Geometry: final body of the model. Coordinates: model frame, mm. Face numbers are marked on the shaded views. A direction names the side the tool comes from. Round coordinates to 2 decimals unless told otherwise and drop trailing zeros. Write each loop counter-clockwise with the first axis right and the second up, starting at its lowest first coordinate (ties: lowest second). Pieces come first, ordered by that corner, then holes.
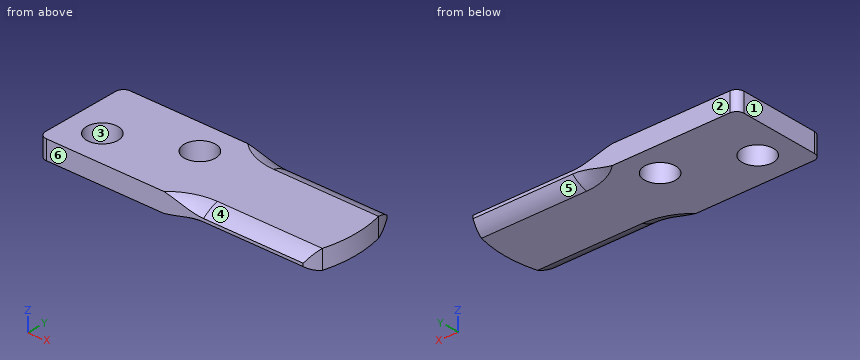
from build123d import *

# Parameters (mm, degrees)
F0_R     = 3.2512
F1_DEPTH = 3.9624


with BuildPart() as f1:
    # F0 (on Top) → F1 (new body)
    with BuildSketch(Plane.XY):
        with BuildLine():
            ThreePointArc((1.5875, 9.8425), (0.464968, 9.377532), (0, 8.255))
            Line((0, 8.255), (0, -8.255))
            ThreePointArc((0, -8.255), (0.464968, -9.377532), (1.5875, -9.8425))
            Line((1.5875, -9.8425), (26.001034, -9.8425))
            ThreePointArc((26.001034, -9.8425), (29.838111, -7.433166), (34.29, -6.5913))
            Line((34.29, -6.5913), (56.127475, -6.5913))
            ThreePointArc((56.127475, -6.5913), (56.9976, 0), (56.127475, 6.5913))
            Line((56.127475, 6.5913), (34.29, 6.5913))
            ThreePointArc((34.29, 6.5913), (29.838111, 7.433166), (26.001034, 9.8425))
            Line((26.001034, 9.8425), (1.5875, 9.8425))
        make_face()
        with Locations((7.0104, -2.8321)):
            Circle(F0_R, mode=Mode.SUBTRACT)
        with Locations((21.9964, 3.1623)):
            Circle(F0_R, mode=Mode.SUBTRACT)
        with BuildLine():
            Line((55.01309, 9.8425), (26.001034, 9.8425))
            ThreePointArc((26.001034, 9.8425), (29.838111, 7.433166), (34.29, 6.5913))
            Line((34.29, 6.5913), (56.127475, 6.5913))
            ThreePointArc((56.127475, 6.5913), (55.625336, 8.23577), (55.01309, 9.8425))
        make_face()
        with BuildLine():
            ThreePointArc((34.29, -6.5913), (29.838111, -7.433166), (26.001034, -9.8425))
            Line((26.001034, -9.8425), (55.01309, -9.8425))
            ThreePointArc((55.01309, -9.8425), (55.625336, -8.23577), (56.127475, -6.5913))
            Line((56.127475, -6.5913), (34.29, -6.5913))
        make_face()
    extrude(amount=F1_DEPTH)

    # F4: sweep along a path in F0
    with BuildLine(Plane.XY) as f4_path:
        Line((60.852341, 6.5913), (34.29, 6.5913))
        ThreePointArc((34.29, 6.5913), (29.838111, 7.433166), (26.001034, 9.8425))
    # F3 (on offset) → F4 (sweep, cut)
    with BuildSketch(Plane.YZ.offset(56.9976)):
        with BuildLine():
            Line((13.0175, 1.6764), (9.8425, 1.6764))
            ThreePointArc((9.8425, 1.6764), (8.313989, 0.649906), (6.5913, 0))
            Line((6.5913, 0), (6.5913, -3.175))
            Line((6.5913, -3.175), (13.0175, -3.175))
            Line((13.0175, -3.175), (13.0175, 1.6764))
        make_face()
        with BuildLine():
            ThreePointArc((6.5913, 3.9624), (8.313989, 3.312494), (9.8425, 2.286))
            Line((9.8425, 2.286), (13.0175, 2.286))
            Line((13.0175, 2.286), (13.0175, 7.1374))
            Line((13.0175, 7.1374), (6.5913, 7.1374))
            Line((6.5913, 7.1374), (6.5913, 3.9624))
        make_face()
    sweep(path=f4_path.line, mode=Mode.SUBTRACT)

    # F5: sweep along a path in F0
    with BuildLine(Plane.XY) as f5_path:
        Line((60.852341, -6.5913), (34.29, -6.5913))
        ThreePointArc((34.29, -6.5913), (29.838111, -7.433166), (26.001034, -9.8425))
    # F3 (on offset) → F5 (sweep, cut)
    with BuildSketch(Plane.YZ.offset(56.9976)):
        with BuildLine():
            Line((-6.5913, -3.175), (-6.5913, 0))
            ThreePointArc((-6.5913, 0), (-8.313989, 0.649906), (-9.8425, 1.6764))
            Line((-9.8425, 1.6764), (-13.02766, 1.6764))
            Line((-13.02766, 1.6764), (-13.02766, -3.175))
            Line((-13.02766, -3.175), (-6.5913, -3.175))
        make_face()
        with BuildLine():
            ThreePointArc((-9.8425, 2.286), (-8.313989, 3.312494), (-6.5913, 3.9624))
            Line((-6.5913, 3.9624), (-6.5913, 7.1374))
            Line((-6.5913, 7.1374), (-13.02766, 7.1374))
            Line((-13.02766, 7.1374), (-13.02766, 2.286))
            Line((-13.02766, 2.286), (-9.8425, 2.286))
        make_face()
    sweep(path=f5_path.line, mode=Mode.SUBTRACT)


solid = f1.part
1) Reachability of the marked faces 4, 5 and 6 from +Z, -Z, +X, -X, +Y, -Y: full face, straight path, thin tool, end or side. Return the list, or none.
2) Section B-B on y = -2. Output: boundary loops of the cut face in (x, z), plus the area to 3 significant figures.
3) Line query: probe 1 along X at (y, z) = (-5.75, 2.1); probe 2 along X at (y, z) = (-3.5, 1); probe 3 along Y at (x, z) = (5.5, 1). Output: solid intervals per line, ascending.
4) Section A-A on x = 8. Output: boundary loops of the cut face in (y, z).
5) Section D-D on x = 41. Output: boundary loops of the cut face in (y, z).
6) Section C-C on z = 3.45. Output: boundary loops of the cut face in (x, y) (1 decimal).
7) Draft query along X for the marked faces 1, 2 and 3. Return one class per face: pulls with the +X half, pulls with the -X half, needs draft (parallel to the pull), parting line crosses it, or undercut.
Filled in:
1. face 4: +Z, +X, -Y
1. face 5: -Z, +X, +Y
1. face 6: +Z, -Z, +X, -X, -Y
2. outline: (0, 0) - (3.87, 0) - (3.87, 3.96) - (0, 3.96) - close; (10.15, 0) - (56.92, 0) - (56.92, 3.96) - (10.15, 3.96) - close
2. area: 201 mm2
3. probe 1: x = 0 to 5.58, 8.44 to 56.34
3. probe 2: x = 0 to 3.83, 10.19 to 56.76
3. probe 3: y = -9.84 to -5.71, 0.05 to 9.84
4. outline: (-9.84, 0) - (-5.93, 0) - (-5.93, 3.96) - (-9.84, 3.96) - close; (0.26, 0) - (9.84, 0) - (9.84, 3.96) - (0.26, 3.96) - close
5. outline: (-9.84, 1.68) arc R8 ccw to (-6.59, 0) - (6.59, 0) arc R8 ccw to (9.84, 1.68) - (9.84, 2.29) arc R8 ccw to (6.59, 3.96) - (-6.59, 3.96) arc R8 ccw to (-9.84, 2.29) - close
6. outline: (0, -8.3) arc R1.6 ccw to (1.6, -9.8) - (28.3, -9.8) arc R10.7 cw to (34.3, -8) - (55.7, -8) arc R25.4 ccw to (56.1, -6.6) arc R25.4 ccw to (56.1, 6.6) arc R25.4 ccw to (55.7, 8) - (34.3, 8) arc R10.7 cw to (28.3, 9.8) - (1.6, 9.8) arc R1.6 ccw to (0, 8.3) - close; hole circle Ø6.5 at (7, -2.8); hole circle Ø6.5 at (22, 3.2)
7. face 1: pulls with the -X half
7. face 2: needs draft
7. face 3: undercut
